Check sheet for the modelled part. Datum: model origin and axes. Units: mm. Face numbers are marked on the shaded views. A direction names the side the tool comes from. Give positions to 0.01 mm unless a question says otherwise; leave off trailing zeros. Order: outer loops, then holes, each group sorted by start corner. A loop starts at its lowest first (then second) coordinate and runs counter-clockwise, first axis right, second up. Notation, with made-up numbers: (-6, 49.5) - (44, 49.5) arc R24 cw to (44, 69.5) - close; hole circle Ø1 at (-6.75, 40). An arc over 180 degrees is marked (long way). Answer in a Markdown table with one row per item.
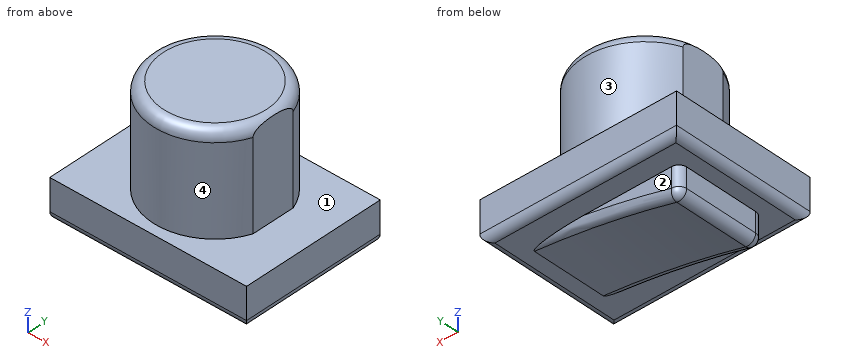
from build123d import *

# Parameters (mm, degrees)
SKETCH1_W               = 11.303
SKETCH1_H               = 4.219764922
BOSS_EXTRUDE1_DEPTH     = 9.6012
SKETCH2_W               = 19.1262
SKETCH2_H               = 14.0462
BOSS_EXTRUDE2_DEPTH     = 3.81
SKETCH3_W               = 14.8082
SKETCH3_H               = 8.763
BOSS_EXTRUDE3_DEPTH     = 2.921
CUT_EXTRUDE1_DEPTH      = 18.711601402
CUT_EXTRUDE1_DEPTH_BACK = 18.711601402
FILLET1_R               = 0.762
FILLET2_R               = 0.762
FILLET3_R               = 0.762
FILLET4_R               = 1.016


with BuildPart() as part:
    # Sketch1 → Boss-Extrude1 (new body)
    with BuildSketch(Plane.XY):
        with BuildLine():
            ThreePointArc((5.6515, 2.109882461), (0, 6.0325), (-5.6515, 2.109882461))
            Line((-5.6515, 2.109882461), (5.6515, 2.109882461))
        make_face()
        Rectangle(SKETCH1_W, SKETCH1_H)
        with BuildLine():
            Line((5.6515, -2.109882461), (-5.6515, -2.109882461))
            ThreePointArc((-5.6515, -2.109882461), (0, -6.0325), (5.6515, -2.109882461))
        make_face()
    extrude(amount=BOSS_EXTRUDE1_DEPTH)

    # Sketch2 → Boss-Extrude2 (add)
    with BuildSketch(Plane(origin=(0, 0, 0), x_dir=(-1, 0, 0), z_dir=(0, 0, -1))):
        Rectangle(SKETCH2_W, SKETCH2_H)
    extrude(amount=BOSS_EXTRUDE2_DEPTH)

    # Sketch3 → Boss-Extrude3 (add)
    with BuildSketch(Plane(origin=(0, 0, -3.81), x_dir=(-1, 0, 0), z_dir=(0, 0, -1))):
        Rectangle(SKETCH3_W, SKETCH3_H)
    extrude(amount=BOSS_EXTRUDE3_DEPTH)

    # Sketch4 → Cut-Extrude1 (cut, two sides: drawn at the far end of the back side and taken through both)
    with BuildSketch(Plane.XZ.offset(4.3815).offset(-CUT_EXTRUDE1_DEPTH_BACK)):
        with BuildLine():
            Line((7.4041, -6.731), (7.4041, -3.81))
            ThreePointArc((7.4041, -3.81), (-0.063420224, -4.948987039), (-7.4041, -6.731))
            Line((-7.4041, -6.731), (7.4041, -6.731))
        make_face()
    extrude(amount=CUT_EXTRUDE1_DEPTH + CUT_EXTRUDE1_DEPTH_BACK, mode=Mode.SUBTRACT)

    # Fillet1
    fillet1_edges = [part.edges().sort_by_distance(p)[0] for p in [
        (-7.4041, 0, -6.731),
    ]]
    fillet(fillet1_edges, radius=FILLET1_R)

    # Fillet2
    fillet2_edges = [part.edges().sort_by_distance(p)[0] for p in [
        (-9.5631, 0, -3.81),
        (0, 7.0231, -3.81),
        (9.5631, 0, -3.81),
        (0, -7.0231, -3.81),
    ]]
    fillet(fillet2_edges, radius=FILLET2_R)

    # Fillet3
    fillet3_edges = [part.edges().sort_by_distance(p)[0] for p in [
        (0.428965251, -4.3815, -4.853334027),
        (0.428965251, 4.3815, -4.853334027),
        (-7.4041, 4.3815, -4.766721364),
        (-7.103485869, 4.3815, -6.329880754),
        (-7.4041, -4.3815, -4.766721364),
        (-7.103485869, -4.3815, -6.329880754),
    ]]
    fillet(fillet3_edges, radius=FILLET3_R)

    # Fillet4
    # the kernel refuses this fillet: 1.016 mm, written as the material it takes off along each edge
    with BuildSketch(Plane(origin=(0, 0, 9.6012), x_dir=(0.9979431218880589, -0.06410558069555868, 0), z_dir=(-0.06410558069555868, -0.9979431218880589, 0))) as fillet4_piece_1:
        with BuildLine():
            CenterArc((6.0325 - FILLET4_R, -FILLET4_R), FILLET4_R, 0, 90)
            Line((6.0325 - FILLET4_R, 0), (6.0325, 0))
            Line((6.0325, 0), (6.0325, -FILLET4_R))
        make_face()
    revolve(axis=Axis((0, 0, 9.6012), (0, 0, 1)), revolution_arc=187.350999162, mode=Mode.SUBTRACT)
    with BuildSketch(Plane(origin=(0, 0, 9.6012), x_dir=(-0.9979431218880589, 0.06410558069555859, 0), z_dir=(0.06410558069555859, 0.9979431218880589, 0))) as fillet4_piece_2:
        with BuildLine():
            CenterArc((6.0325 - FILLET4_R, -FILLET4_R), FILLET4_R, 0, 90)
            Line((6.0325 - FILLET4_R, 0), (6.0325, 0))
            Line((6.0325, 0), (6.0325, -FILLET4_R))
        make_face()
    revolve(axis=Axis((0, 0, 9.6012), (0, 0, 1)), revolution_arc=187.350999162, mode=Mode.SUBTRACT)


solid = part.part
(1) Access from +Z, -Z, +X, -X, +Y, -Y to the whole of each face (thin tool, end or side, straight path). Record for the marked faces 1, 2, 3 and 4.
Geometry says:
| item | result |
|---|---|
| face 1 | +Z |
| face 2 | -Z, +X, -X, +Y |
| face 3 | +Z, +Y |
| face 4 | +Z, -Y |
(2) Thickness scan on L1, parallel to Z at x = -3.75, y = 5.75; L2, parallel to Z at x = -0.25, y = -5; L3, parallel to X at y = -5.5, z = 1.75. Record the ranges inside material, lowest first.
Geometry says:
| item | result |
|---|---|
| L1 | -3.81 to 0 |
| L2 | -3.81 to 9.6 |
| L3 | -2.48 to 2.48 |
(3) Cross-section at B-B, the plane x = -8.5. Record the cut outline in (y, z).
Geometry says:
| item | result |
|---|---|
| outline | (-7.02, -3.05) arc R0.76 ccw to (-6.26, -3.81) - (6.26, -3.81) arc R0.76 ccw to (7.02, -3.05) - (7.02, 0) - (-7.02, 0) - close |
(4) Gauge pin test, flat ends, axial feed: P1, Ø4, axis at x = -3, y = 0.5, coming from the -Z side; P2, Ø1.5, axis at x = -3.5, z = -5, coming from the +Y side; P3, Ø1.5, axis at x = -3, z = -5, coming from the -Y side. Record the tip position at first contact, or that the pin passes through.
Geometry says:
| item | result |
|---|---|
| P1 | z = -6.07 |
| P2 | y = 4.38 |
| P3 | y = -4.38 |
